Build history of the part. All positions in model axes, mm. Face numbers are marked on the shaded views. Coordinates: 2 decimals unless noted, no trailing zeros. Write each loop counter-clockwise with the first axis right and the second up, starting at its lowest first coordinate (ties: lowest second). Pieces come first, ordered by that corner, then holes.
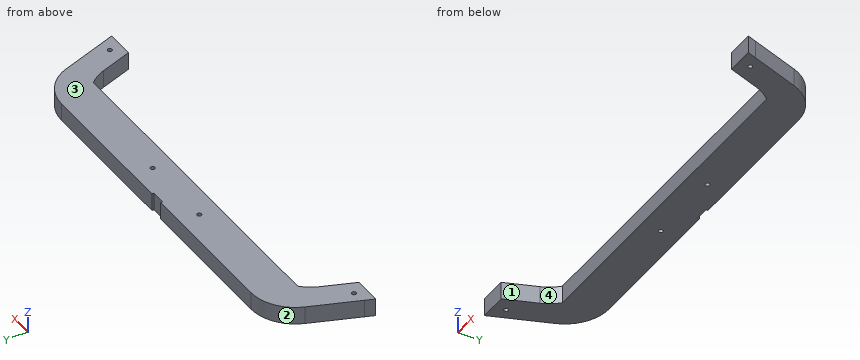
```python
from build123d import *

# Parameters (mm, degrees)
SALIENTE_EXTRUIR1_DEPTH = 40
REDONDEO1_R             = 100
ESCALA1_SCALE           = 0.6
ESCALA2_SCALE           = 0.75
SALIENTE_EXTRUIR2_DEPTH = 18
CROQUIS3_W              = 15
CROQUIS3_H              = 2
CORTAR_EXTRUIR1_DEPTH   = 19
CROQUIS4_R              = 2.25
CORTAR_EXTRUIR3_DEPTH   = 19
CROQUIS5_R              = 2.25
CORTAR_EXTRUIR4_DEPTH   = 19


with BuildPart() as part:
    # Croquis1 → Saliente-Extruir1 (new body)
    with BuildSketch(Plane.XY):
        Polygon((-439, 0), (-388.899497253, 137.65), (388.899497253, 137.65), (439, 0), (502.850666349, 0), (495.381557247, 20.5212086), (430.911949546, 197.65), (-430.911949546, 197.65), (-495.381557247, 20.5212086), (-502.850666349, 0), align=None)
    extrude(amount=SALIENTE_EXTRUIR1_DEPTH)

    # Redondeo1
    redondeo1_edges = [part.edges().sort_by_distance(p)[0] for p in [
        (-430.911949546, 197.65, 20),
        (430.911949546, 197.65, 20),
        (388.899497253, 137.65, 20),
        (-388.899497253, 137.65, 20),
    ]]
    fillet(redondeo1_edges, radius=REDONDEO1_R)


with BuildPart() as part_1:
    # Escala1: scaled about (0, 141.339436806, 20)
    add(part.part.scale(ESCALA1_SCALE).moved(Location((0, 56.535774722, 8))))


with BuildPart() as part_2:
    # Escala2: scaled about (0, 141.339436806, 20)
    add(part_1.part.scale(ESCALA2_SCALE).moved(Location((0, 35.334859202, 5))))

    # Croquis2 → Saliente-Extruir2 (add, through all)
    with BuildSketch(Plane.XY.offset(29)):
        with BuildLine():
            Line((-111.856850505, 126.679190243), (111.856850505, 126.679190243))
            Line((111.856850505, 126.679190243), (175.134018584, 126.679190243))
            ThreePointArc((175.134018584, 126.679190243), (160.598065921, 136.30250102), (143.495434545, 139.679190243))
            Line((143.495434545, 139.679190243), (-143.495434545, 139.679190243))
            ThreePointArc((-143.495434545, 139.679190243), (-160.598065921, 136.30250102), (-175.134018584, 126.679190243))
            Line((-175.134018584, 126.679190243), (-111.856850505, 126.679190243))
        make_face()
    extrude(amount=-SALIENTE_EXTRUIR2_DEPTH)

    # Croquis3 → Cortar-Extruir1 (cut, through all)
    with BuildSketch(Plane.XY.offset(29)):
        with Locations((0, 165.679190243)):
            Rectangle(CROQUIS3_W, CROQUIS3_H)
    extrude(amount=-CORTAR_EXTRUIR1_DEPTH, mode=Mode.SUBTRACT)

    # Croquis4 → Cortar-Extruir3 (cut, through all)
    with BuildSketch(Plane.XY.offset(29)):
        with Locations((209.25, 89.736690243)):
            Circle(CROQUIS4_R)
        with Locations((-209.25, 89.736690243)):
            Circle(CROQUIS4_R)
    extrude(amount=-CORTAR_EXTRUIR3_DEPTH, mode=Mode.SUBTRACT)

    # Croquis5 → Cortar-Extruir4 (cut, through all)
    with BuildSketch(Plane.XY.offset(29)):
        with Locations((-40, 146.679190243)):
            Circle(CROQUIS5_R)
        with Locations((40, 146.679190243)):
            Circle(CROQUIS5_R)
    extrude(amount=-CORTAR_EXTRUIR4_DEPTH, mode=Mode.SUBTRACT)


solid = part_2.part
```
1. Flat gauge pins, fed straight in: pin 1 (8 mm diameter, centred on x = 81, z = 20.5, fed in from -Y); pin 2 (1 mm diameter, centred on y = 99.5, z = 18.5, fed in from +X); pin 3 (1 mm diameter, centred on y = 88.5, z = 22.5, fed in from +X). Where does each tip first touch, or does it go through?
Computed values:
pin 1: stops at y = 126.68
pin 2: stops at x = 218.54
pin 3: stops at x = 222.55
2. Saw through at C-C on y = 132. List the corners of the cut face in (x, z), plus the area to 3 significant figures.
Computed values:
outline: (-206.53, 11) - (206.53, 11) - (206.53, 29) - (-206.53, 29) - close
area: 7,440 mm2
3. Mould opens along X. For the marked faces 1, 2, 3 and 4 say: +X half, -X half, draft (parallel to the pull), parting line (faces both ways), or undercut.
Computed values:
face 1: undercut
face 2: -X half
face 3: draft
face 4: undercut
4. Saw through at A-A on z = 21. List the corners of the cut face in (x, y), plus the area to 3 significant figures.
Computed values:
outline: (-226.28, 77.74) - (-197.55, 77.74) - (-185.78, 110.07) arc R45 cw to (-175.13, 126.68) - (175.13, 126.68) arc R45 cw to (185.78, 110.07) - (197.55, 77.74) - (226.28, 77.74) - (204.69, 137.07) arc R45 ccw to (162.4, 166.68) - (7.5, 166.68) - (7.5, 164.68) - (-7.5, 164.68) - (-7.5, 166.68) - (-162.4, 166.68) arc R45 ccw to (-204.69, 137.07) - close; hole circle Ø4.5 at (-209.25, 89.74); hole circle Ø4.5 at (-40, 146.68); hole circle Ø4.5 at (40, 146.68); hole circle Ø4.5 at (209.25, 89.74)
area: 18,500 mm2
5. Probe line 1 along Y through (x, z) = (40, 22.5); line 2 along X through (y, z) = (88, 25.75); line 3 along Y through (x, z) = (35, 22). List the from-to ranges inside material, lowest first.
Computed values:
line 1: y = 126.68 to 144.43, 148.93 to 166.68
line 2: x = -222.55 to -210.68, -207.82 to -193.81, 193.81 to 207.82, 210.68 to 222.55
line 3: y = 126.68 to 166.68
6. Saw through at B-B on x = 67.5. List the corners of the cut face in (y, z), plus the area to 3 significant figures.
Computed values:
outline: (126.68, 11) - (166.68, 11) - (166.68, 29) - (126.68, 29) - close
area: 720 mm2
